from build123d import *

# Parameters (mm, degrees)
F0_W     = 0.8
F0_H     = 0.8
F1_DEPTH = 8.595
F2_R     = 1.4
F3_DEPTH = 2


with BuildPart() as f1:
    # F0 (on Top) → F1 (new body, symmetric)
    with BuildSketch(Plane.XY):
        with Locations((8.25, 9.6)):
            Rectangle(F0_W, F0_H)
        Polygon((8.65, 9.2), (8.65, 2), (10.25, 2), (10.25, 10), (8.65, 10), align=None)
        with Locations((-8.25, 9.6)):
            Rectangle(F0_W, F0_H)
        Polygon((-10.25, 10), (-10.25, 2), (-8.65, 2), (-8.65, 9.2), (-8.65, 10), align=None)
        Polygon((-10.25, 0), (0, 0), (0, 2), (-8.65, 2), (-10.25, 2), align=None)
        Polygon((0, 2), (0, 0), (10.25, 0), (10.25, 2), (8.65, 2), align=None)
    extrude(amount=F1_DEPTH, both=True)

    # F2 (on face) → F3 (cut, through all)
    with BuildSketch(Plane.XZ):
        Circle(F2_R)
    extrude(amount=-F3_DEPTH, mode=Mode.SUBTRACT)


solid = f1.part
Source: CAD feature listing. Evaluate the final solid. Frame: model axes, mm. A direction names the side the tool comes from. Round coordinates to 2 decimals unless told otherwise and drop trailing zeros. Loops run counter-clockwise (first coordinate to the right, second up) from the corner with the lowest first, then second, coordinate; pieces in that order, holes last. Notation, with made-up numbers: (63.25, -37.5) -> (103.25, -37.5) arc R26 cw to (103.25, -9.5) -> close; hole circle Ø4 at (16.5, -8). An arc over 180 degrees is marked (long way). Answer as a JSON object with one key per item and string values. Group by question number.
Q1. Section query C-C (y = 9.5). Output: boundary loops of the cut face in (x, z) (3 decimals), plus the area to 3 significant figures.
Q2. Section query D-D (z = -2). Output: boundary loops of the cut face in (x, y).
Q3. Ray query, line 1 (Z direction, x = 0, y = 1.3) (3 decimals); line 2 (X direction, y = 6.75, z = -6.25); line 3 (Y direction, x = -5.25, z = 0.5). Return the intervals inside material, ascending. Write a range as from..to.
Q4. Section query A-A (x = 0). Output: boundary loops of the cut face in (y, z) (3 decimals).
Q5. Access query for faces 4 (the flat face through (-8.65, 6, 0)), 5 (the flat face through (0, 0, 2)), 6 (the flat face through (7.85, 9.6, 0.1)). Directions: +Z, -Z, +X, -X, +Y, -Y. A direction counts if a zero-diameter tool reaches every point of the face in a straight line with its end or side. Return the directions, or none.
Q6. Contact query for a flat-ended pin moving along its axis: P1, Ø4, axis at x = -3, z = -2.5, coming from the +Y side. Output: stop coordinate, or through.
Q7. Mould query, pull axis X, two halves, no side actions, for faces 1 (the flat face through (9, 10, 0)), 2 (the flat face through (10.25, 5, 0)), 3 (the flat face through (-7.85, 9.6, 0.1)). Classes: pulls with the +X half, pulls with the -X half, needs draft (parallel to the pull), parting line crosses it, or undercut.
Q8. Section query B-B (z = 0). Output: boundary loops of the cut face in (x, y), plus the area to 3 significant figures.
Completed:
{
 "1": {"outline": "(-10.25, -8.595) -> (-7.85, -8.595) -> (-7.85, 8.595) -> (-10.25, 8.595) -> close; (7.85, -8.595) -> (10.25, -8.595) -> (10.25, 8.595) -> (7.85, 8.595) -> close", "area": "82.5 mm²"},
 "2": {"outline": "(-10.25, 0) -> (10.25, 0) -> (10.25, 10) -> (7.85, 10) -> (7.85, 9.2) -> (8.65, 9.2) -> (8.65, 2) -> (-8.65, 2) -> (-8.65, 9.2) -> (-7.85, 9.2) -> (-7.85, 10) -> (-10.25, 10) -> close"},
 "3": {"line 1": "-8.595..-1.4, 1.4..8.595", "line 2": "-10.25..-8.65, 8.65..10.25", "line 3": "0..2"},
 "4": {"outline": "(0, -8.595) -> (2, -8.595) -> (2, -1.4) -> (0, -1.4) -> close; (0, 1.4) -> (2, 1.4) -> (2, 8.595) -> (0, 8.595) -> close"},
 "5": {"face 4": "+Z, -Z", "face 5": "+Z, -Z, +X, -X, -Y", "face 6": "+Z, -Z, +Y"},
 "6": {"P1": "y = 2"},
 "7": {"face 1": "needs draft", "face 2": "pulls with the +X half", "face 3": "undercut"},
 "8": {"outline": "(-10.25, 0) -> (-1.4, 0) -> (-1.4, 2) -> (-8.65, 2) -> (-8.65, 9.2) -> (-7.85, 9.2) -> (-7.85, 10) -> (-10.25, 10) -> close; (1.4, 0) -> (10.25, 0) -> (10.25, 10) -> (7.85, 10) -> (7.85, 9.2) -> (8.65, 9.2) -> (8.65, 2) -> (1.4, 2) -> close", "area": "62.3 mm²"}
}
